from build123d import *

# Parameters (mm, degrees)
SKETCH1_W           = 45
SKETCH1_H           = 10
BOSS_EXTRUDE1_DEPTH = 5
SKETCH3_R           = 1.5
SKETCH3_R_2         = 2.175
SKETCH3_R_3         = 1.75
CUT_EXTRUDE1_DEPTH  = 7
FILLET1_R           = 2
SKETCH4_R           = 3
SKETCH4_R_2         = 1.5
BOSS_EXTRUDE2_DEPTH = 2.5
SKETCH5_W           = 10
SKETCH5_H           = 5
BOSS_EXTRUDE3_DEPTH = 19
SKETCH6_R           = 1.5
CUT_EXTRUDE2_DEPTH  = 10
BOSS_EXTRUDE4_START = 2
SKETCH7_R           = 3
SKETCH7_R_2         = 1.5
BOSS_EXTRUDE4_DEPTH = 2
FILLET2_R           = 7
CHAMFER1_SIZE       = 1


with BuildPart() as part:
    # Sketch1 → Boss-Extrude1 (new body)
    with BuildSketch(Plane(origin=(0, 0, 0), x_dir=(1, 0, 0), z_dir=(0, 1, 0))):
        Rectangle(SKETCH1_W, SKETCH1_H)
    extrude(amount=BOSS_EXTRUDE1_DEPTH)

    # Sketch3 → Cut-Extrude1 (cut)
    with BuildSketch(Plane(origin=(0, 5, 0), x_dir=(1, 0, 0), z_dir=(0, 1, 0))):
        with Locations(Location((-18.55, 0, 0), (0, 0, 270))):
            Circle(SKETCH3_R)
        with Locations(Location((9.5, 0, 0), (0, 0, 270))):
            Circle(SKETCH3_R_2)
        with Locations(Location((-6.55, 0, 0), (0, 0, 270))):
            Circle(SKETCH3_R_3)
        with Locations(Location((17.45, 0, 0), (0, 0, 270))):
            Circle(SKETCH3_R_3)
    extrude(amount=-CUT_EXTRUDE1_DEPTH, mode=Mode.SUBTRACT)

    # Fillet1
    fillet1_edges = [part.edges().sort_by_distance(p)[0] for p in [
        (22.5, 2.5, 5),
        (-22.5, 2.5, 5),
        (-22.5, 2.5, -5),
        (22.5, 2.5, -5),
    ]]
    fillet(fillet1_edges, radius=FILLET1_R)

    # Sketch4 → Boss-Extrude2 (add)
    with BuildSketch(Plane.XZ):
        with Locations(Location((-18.55, 0, 0), (0, 0, 270))):
            Circle(SKETCH4_R)
        with Locations(Location((-18.55, 0, 0), (0, 0, 90))):
            Circle(SKETCH4_R_2, mode=Mode.SUBTRACT)
    extrude(amount=BOSS_EXTRUDE2_DEPTH)

    # Sketch5 → Boss-Extrude3 (add)
    with BuildSketch(Plane(origin=(0, 0, -5), x_dir=(-1, 0, 0), z_dir=(0, 0, -1))):
        with Locations((-9.5, 2.5)):
            Rectangle(SKETCH5_W, SKETCH5_H)
    extrude(amount=BOSS_EXTRUDE3_DEPTH)

    # Sketch6 → Cut-Extrude2 (cut)
    with BuildSketch(Plane(origin=(0, 5, 0), x_dir=(1, 0, 0), z_dir=(0, 1, 0))):
        with Locations(Location((9.5, 19.5, 0), (0, 0, 270))):
            Circle(SKETCH6_R)
    extrude(amount=-CUT_EXTRUDE2_DEPTH, mode=Mode.SUBTRACT)

    # Sketch7 → Boss-Extrude4 (add)
    with BuildSketch(Plane(origin=(0, 5, 0), x_dir=(1, 0, 0), z_dir=(0, 1, 0)).offset(BOSS_EXTRUDE4_START)):
        with Locations(Location((9.5, 19.5, 0), (0, 0, 270))):
            Circle(SKETCH7_R)
        with Locations(Location((9.5, 19.5, 0), (0, 0, 270))):
            Circle(SKETCH7_R_2, mode=Mode.SUBTRACT)
    extrude(amount=-BOSS_EXTRUDE4_DEPTH)

    # Fillet2
    fillet2_edges = [part.edges().sort_by_distance(p)[0] for p in [
        (4.5, 2.5, -5),
        (14.5, 2.5, -5),
    ]]
    fillet(fillet2_edges, radius=FILLET2_R)

    # Chamfer1
    # the kernel refuses this chamfer: 1 mm, written as the material it takes off along each edge
    with BuildSketch(Plane(origin=(-20.5, 0, -5), x_dir=(0, 1, 0), z_dir=(1, 0, 0))) as chamfer1_piece_1:
        Polygon((CHAMFER1_SIZE, 0), (0, CHAMFER1_SIZE), (0, 0), align=None)
    extrude(amount=18, mode=Mode.SUBTRACT)
    with BuildSketch(Plane(origin=(-20.5, 5, -5), x_dir=(0, -1, 0), z_dir=(1, 0, 0))) as chamfer1_piece_2:
        Polygon((CHAMFER1_SIZE, 0), (0, -CHAMFER1_SIZE), (0, 0), align=None)
    extrude(amount=18, mode=Mode.SUBTRACT)
    with BuildSketch(Plane(origin=(20.5, 0, -3), x_dir=(0.11111111111111072, 0, -0.9938079899999066), z_dir=(-0.9938079899999066, 0, -0.11111111111111072))) as chamfer1_piece_3:
        Polygon((2 - CHAMFER1_SIZE, 0), (2, -CHAMFER1_SIZE), (2, 0), align=None)
    revolve(axis=Axis((20.5, 0, -3), (0, -1, 0)), revolution_arc=83.620629792, mode=Mode.SUBTRACT)
    with BuildSketch(Plane(origin=(-2.5, 5, -12), x_dir=(0, 0, 1), z_dir=(-1, 0, 0))) as chamfer1_piece_4:
        Polygon((7, -CHAMFER1_SIZE), (7 + CHAMFER1_SIZE, 0), (7, 0), align=None)
    revolve(axis=Axis((-2.5, 5, -12), (0, 1, 0)), revolution_arc=90, mode=Mode.SUBTRACT)
    with BuildSketch(Plane(origin=(-2.5, 0, -12), x_dir=(0, 0, 1), z_dir=(-1, 0, 0))) as chamfer1_piece_5:
        Polygon((7 + CHAMFER1_SIZE, 0), (7, CHAMFER1_SIZE), (7, 0), align=None)
    revolve(axis=Axis((-2.5, 0, -12), (0, 1, 0)), revolution_arc=90, mode=Mode.SUBTRACT)
    with BuildSketch(Plane(origin=(21.499999975, 0, -11.944271843), x_dir=(-0.11111110870133047, 0, 0.9938079902693282), z_dir=(0.9938079902693282, 0, 0.11111110870133047))) as chamfer1_piece_6:
        Polygon((6.999999931 + CHAMFER1_SIZE, 0), (6.999999931 + CHAMFER1_SIZE * 6.29164365051e-09, -CHAMFER1_SIZE), (6.999999931, 0), align=None)
    revolve(axis=Axis((21.499999975, 0, -11.944271843), (0, -1, 0)), revolution_arc=83.620630478, mode=Mode.SUBTRACT)
    with BuildSketch(Plane(origin=(21.499999975, 5, -11.944271843), x_dir=(-0.11111110870132958, 0, 0.9938079902693283), z_dir=(0.9938079902693283, 0, 0.11111110870132958))) as chamfer1_piece_7:
        Polygon((6.999999931 + CHAMFER1_SIZE, 0), (6.999999931 + CHAMFER1_SIZE * 6.2916400978e-09, CHAMFER1_SIZE), (6.999999931, 0), align=None)
    revolve(axis=Axis((21.499999975, 5, -11.944271843), (0, -1, 0)), revolution_arc=83.620630478, mode=Mode.SUBTRACT)
    with BuildSketch(Plane(origin=(22.5, 0, -3), x_dir=(-1, 0, 0), z_dir=(0, 0, 1))) as chamfer1_piece_8:
        Polygon((CHAMFER1_SIZE, 0), (0, -CHAMFER1_SIZE), (0, 0), align=None)
    extrude(amount=6, mode=Mode.SUBTRACT)
    with BuildSketch(Plane(origin=(20.5, 0, 5), x_dir=(0, 0, -1), z_dir=(-1, 0, 0))) as chamfer1_piece_9:
        Polygon((CHAMFER1_SIZE, 0), (0, -CHAMFER1_SIZE), (0, 0), align=None)
    extrude(amount=41, mode=Mode.SUBTRACT)
    with BuildSketch(Plane(origin=(-22.5, 0, 3), x_dir=(1, 0, 0), z_dir=(0, 0, -1))) as chamfer1_piece_10_section:
        Polygon((CHAMFER1_SIZE, 0), (0, -CHAMFER1_SIZE), (0, 0), align=None)
    chamfer1_piece_10 = extrude(amount=6, mode=Mode.PRIVATE)
    chamfer1_piece_10 = chamfer1_piece_10 - Plane(origin=(-18.55, 0, 0), x_dir=(0, 0, -1), z_dir=(0, 1, 0)) * Cylinder(3, 16, mode=Mode.PRIVATE)
    add(chamfer1_piece_10, mode=Mode.SUBTRACT)
    with BuildSketch(Plane(origin=(-20.5, 0, 3), x_dir=(-1, 0, 0), z_dir=(0, 0, -1))) as chamfer1_piece_11:
        Polygon((2 - CHAMFER1_SIZE, 0), (2, CHAMFER1_SIZE), (2, 0), align=None)
    revolve(axis=Axis((-20.5, 0, 3), (0, 1, 0)), revolution_arc=90, mode=Mode.SUBTRACT)
    with BuildSketch(Plane(origin=(20.5, 0, 3), x_dir=(1, 0, 0), z_dir=(0, 0, -1))) as chamfer1_piece_12:
        Polygon((2 - CHAMFER1_SIZE, 0), (2, -CHAMFER1_SIZE), (2, 0), align=None)
    revolve(axis=Axis((20.5, 0, 3), (0, -1, 0)), revolution_arc=90, mode=Mode.SUBTRACT)
    with BuildSketch(Plane(origin=(-20.5, 0, -3), x_dir=(0, 0, -1), z_dir=(1, 0, 0))) as chamfer1_piece_13:
        Polygon((2 - CHAMFER1_SIZE, 0), (2, CHAMFER1_SIZE), (2, 0), align=None)
    revolve(axis=Axis((-20.5, 0, -3), (0, 1, 0)), revolution_arc=90, mode=Mode.SUBTRACT)
    with BuildSketch(Plane(origin=(22.5, 5, -3), x_dir=(-1, 0, 0), z_dir=(0, 0, 1)), Plane(origin=(-22.5, 5, 3), x_dir=(1, 0, 0), z_dir=(0, 0, -1))) as chamfer1_piece_14:
        Polygon((CHAMFER1_SIZE, 0), (0, CHAMFER1_SIZE), (0, 0), align=None)
    extrude(amount=6, mode=Mode.SUBTRACT)
    with BuildSketch(Plane(origin=(20.5, 5, 5), x_dir=(0, 0, -1), z_dir=(-1, 0, 0))) as chamfer1_piece_15:
        Polygon((CHAMFER1_SIZE, 0), (0, CHAMFER1_SIZE), (0, 0), align=None)
    extrude(amount=41, mode=Mode.SUBTRACT)
    with BuildSketch(Plane(origin=(-20.5, 5, 3), x_dir=(-1, 0, 0), z_dir=(0, 0, -1))) as chamfer1_piece_16:
        Polygon((2 - CHAMFER1_SIZE, 0), (2, -CHAMFER1_SIZE), (2, 0), align=None)
    revolve(axis=Axis((-20.5, 5, 3), (0, 1, 0)), revolution_arc=90, mode=Mode.SUBTRACT)
    with BuildSketch(Plane(origin=(20.5, 5, 3), x_dir=(1, 0, 0), z_dir=(0, 0, -1))) as chamfer1_piece_17:
        Polygon((2 - CHAMFER1_SIZE, 0), (2, CHAMFER1_SIZE), (2, 0), align=None)
    revolve(axis=Axis((20.5, 5, 3), (0, -1, 0)), revolution_arc=90, mode=Mode.SUBTRACT)
    with BuildSketch(Plane(origin=(-20.5, 5, -3), x_dir=(0, 0, -1), z_dir=(1, 0, 0))) as chamfer1_piece_18:
        Polygon((2, -CHAMFER1_SIZE), (2 - CHAMFER1_SIZE, 0), (2, 0), align=None)
    revolve(axis=Axis((-20.5, 5, -3), (0, 1, 0)), revolution_arc=90, mode=Mode.SUBTRACT)
    with BuildSketch(Plane(origin=(20.5, 5, -3), x_dir=(0.11111111111111072, 0, -0.9938079899999066), z_dir=(-0.9938079899999066, 0, -0.11111111111111072))) as chamfer1_piece_19:
        Polygon((2 - CHAMFER1_SIZE, 0), (2, CHAMFER1_SIZE), (2, 0), align=None)
    revolve(axis=Axis((20.5, 5, -3), (0, -1, 0)), revolution_arc=83.620629792, mode=Mode.SUBTRACT)
    with BuildSketch(Plane(origin=(14.5, 5, -11.94427191), x_dir=(-1, 0, 0), z_dir=(0, 0, -1))) as chamfer1_piece_20:
        Polygon((CHAMFER1_SIZE, 0), (0, -CHAMFER1_SIZE), (0, 0), align=None)
    extrude(amount=14.627411078, mode=Mode.SUBTRACT)
    with BuildSketch(Plane(origin=(14.5, 0, -11.94427191), x_dir=(-1, 0, 0), z_dir=(0, 0, -1))) as chamfer1_piece_21:
        Polygon((CHAMFER1_SIZE, 0), (0, CHAMFER1_SIZE), (0, 0), align=None)
    extrude(amount=14.627411078, mode=Mode.SUBTRACT)
    with BuildSketch(Plane(origin=(4.5, 0, -12), x_dir=(1, 0, 0), z_dir=(0, 0, -1))) as chamfer1_piece_22:
        Polygon((CHAMFER1_SIZE, 0), (0, -CHAMFER1_SIZE), (0, 0), align=None)
    extrude(amount=14.571682988, mode=Mode.SUBTRACT)
    with BuildSketch(Plane(origin=(4.5, 5, -12), x_dir=(1, 0, 0), z_dir=(0, 0, -1))) as chamfer1_piece_23:
        Polygon((CHAMFER1_SIZE, 0), (0, CHAMFER1_SIZE), (0, 0), align=None)
    extrude(amount=14.571682988, mode=Mode.SUBTRACT)


solid = part.part
Work out the finished part from the listing and answer in its coordinate system (mm). A direction names the side the tool comes from. Coordinates: 2 decimals unless noted, no trailing zeros. Loops run counter-clockwise (first coordinate to the right, second up) from the corner with the lowest first, then second, coordinate; pieces in that order, holes last. Notation, with made-up numbers: (12, 64) -> (56, 64) arc R20 ccw to (56, 93) -> close; hole circle Ø10 at (19.25, 82.5). An arc over 180 degrees is marked (long way). Answer as CSV lines item,"result".
1) The part is cut by section B-B (x = 9.5). Give the vertices of the cut face in (y, z) (3 decimals).
A:
outline,"(0, -24) -> (5, -24) -> (5, -22.5) -> (7, -22.5) -> (7, -21) -> (0, -21) -> close; (0, -18) -> (7, -18) -> (7, -16.5) -> (5, -16.5) -> (5, -2.175) -> (0, -2.175) -> close; (0, 2.175) -> (5, 2.175) -> (5, 4) -> (4, 5) -> (1, 5) -> (0, 4) -> close"
2) The part is cut by section A-A (x = -6.55). Give the vertices of the cut face in (y, z), and give its area (3 significant figures).
A:
outline,"(0, -4) -> (1, -5) -> (4, -5) -> (5, -4) -> (5, -1.75) -> (0, -1.75) -> close; (0, 1.75) -> (5, 1.75) -> (5, 4) -> (4, 5) -> (1, 5) -> (0, 4) -> close"
area,"30.5 mm²"
3) For a pull along X with two mould halves and no side action, classify faces 4 (the face through (-8.1, 2.54, 0.81)), 5 (the face through (19.185, 2.535, -0.228)), 6 (the face through (21.9, 2.52, 4.43)), 7 (the face through (-21.5, 0.4, 3.98)) as released by +X, released by -X, zero draft, split by the parting line, or undercut.
A:
face 4,"undercut"
face 5,"undercut"
face 6,"released by +X"
face 7,"released by -X"
4) The part is cut by section C-C (z = -19.5). Give the vertices of the cut face in (x, y), and give its area (3 significant figures).
A:
outline,"(4.5, 1) -> (5.5, 0) -> (8, 0) -> (8, 7) -> (6.5, 7) -> (6.5, 5) -> (5.5, 5) -> (4.5, 4) -> close; (11, 0) -> (13.5, 0) -> (14.5, 1) -> (14.5, 4) -> (13.5, 5) -> (12.5, 5) -> (12.5, 7) -> (11, 7) -> close"
area,"39.0 mm²"
5) Straight lines are drawn through the part: probe 1 along X at (y, z) = (3.8, 0) (3 decimals); probe 2 along Y at (x, z) = (11, -4); probe 3 along X at (y, z) = (4.75, 0) (3 decimals). For each, find the intervals that lie inside material, in ascending order.
A:
probe 1,"x = -22.5 to -20.05, -17.05 to -8.3, -4.8 to 7.325, 11.675 to 15.7, 19.2 to 22.5"
probe 2,"y = 0 to 5"
probe 3,"x = -21.75 to -20.05, -17.05 to -8.3, -4.8 to 7.325, 11.675 to 15.7, 19.2 to 21.75"
6) The part is cut by section D-D (y = 2.25). State how many separate pieces and enclosed holes the cut face has, and give its area (3 significant figures).
A:
separate pieces,"1"
enclosed holes,"5"
area,"609 mm²"
7) Flat-ended cylindrical pins translate along their axes: pin 1 (0.9 mm diameter, centred on y = 2.5, z = -16, fed in from +X); pin 2 (3.5 mm diameter, centred on x = 9.5, z = 0, fed in from +Y); pin 3 (5.5 mm diameter, centred on x = 17.45, z = 0, fed in from +Y); pin 4 (3.5 mm diameter, centred on x = -15.5, y = 3, fed in from -Z). Find the tip coordinate at first contact, or state that the pin passes through.
A:
pin 1,"stops at x = 14.5"
pin 2,"passes through"
pin 3,"stops at y = 5"
pin 4,"stops at z = -5"
8) For faces 1 (the face through (14, 0.5, -17.9)), 2 (the face through (-11.6, 0.5, -4.5)), 3 (the face through (-11.6, 4.5, -4.5)), determine the directions among +Z, -Z, +X, -X, +Y, -Y from which every point of the face is accessible in a straight line to the end or side of a thin tool.
A:
face 1,"-Z, +X, -Y"
face 2,"-Z, -X, -Y"
face 3,"-Z, -X, +Y"
